from build123d import *

# Parameters (mm, degrees)
F0_W     = 3.8
F0_H     = 5
F0_W_2   = 4
F0_H_2   = 4
F0_R     = 2.5006647493
F0_R_2   = 4.8327220748
F0_R_3   = 3.906097333
F0_R_4   = 2.1231290944
F0_R_5   = 7.6831288046
F0_W_3   = 12
F0_H_3   = 6
F0_R_6   = 1.5
F1_DEPTH = 7
F2_SIZE  = 0.75


# Not quite as in the source:
# - a feature names something its author has since deleted; it is built from what else it names


with BuildPart() as f1:
    # F0 (on Top) → F1 (new body)
    with BuildSketch(Plane.XY):
        Polygon((0, 10.6260057762), (0, 15.6260057762), (-4, 15.6260057762), (-4, -26.3739942238), (0, -26.3739942238), (0, -22.3739942238), align=None)
        Polygon((8, 15.6260057762), (0, 15.6260057762), (0, 10.6260057762), (4.2, 10.6260057762), (8, 10.6260057762), align=None)
        with Locations((6.1, 8.1260057762)):
            Rectangle(F0_W, F0_H)
        with Locations((2, -24.3739942238)):
            Rectangle(F0_W_2, F0_H_2)
        Polygon((-4, -26.3739942238), (-4, 15.6260057762), (-42, 15.6260057762), (-42, 9.6260057762), (-54, 9.6260057762), align=None)
        with Locations((-21.8336265534, -6.3459714875)):
            Circle(F0_R, mode=Mode.SUBTRACT)
        with Locations((-12.1693955734, -9.9561735988)):
            Circle(F0_R_2, mode=Mode.SUBTRACT)
        with Locations((-28.6096986383, 0.2079327387)):
            Circle(F0_R, mode=Mode.SUBTRACT)
        with Locations((-36.4965982735, 7.095086854)):
            Circle(F0_R_3, mode=Mode.SUBTRACT)
        with Locations((-27.8876554221, 10.2054132149)):
            Circle(F0_R_4, mode=Mode.SUBTRACT)
        with Locations((-16.008509323, 5.6881718338)):
            Circle(F0_R_5, mode=Mode.SUBTRACT)
        with Locations((-48, 12.6260057762)):
            Rectangle(F0_W_3, F0_H_3)
        with Locations((-51, 12.6260057762)):
            Circle(F0_R_6, mode=Mode.SUBTRACT)
        with Locations((-45, 12.6260057762)):
            Circle(F0_R_6, mode=Mode.SUBTRACT)
    extrude(amount=F1_DEPTH)

    # F2
    f2_edges = [f1.edges().sort_by_distance(p)[0] for p in [
        (4.2, 5.626006, 3.5),
        (4, -22.373994, 3.5),
        (-17.002118, -9.956174, 0),
        (-31.110363, 0.207933, 0),
        (-40.402696, 7.095087, 7),
        (-40.402696, 7.095087, 0),
        (-30.010785, 10.205413, 0),
        (-23.691638, 5.688172, 0),
        (0, -5.873994, 0),
        (2.1, 10.626006, 0),
        (4.2, 8.126006, 0),
        (6.1, 5.626006, 0),
        (8, 10.626006, 0),
        (-23, 15.626006, 0),
        (-54, 12.626006, 0),
        (-29, -8.373994, 0),
        (0, -26.373994, 0),
        (4, -24.373994, 0),
        (2, -22.373994, 0),
        (-23, 15.626006, 7),
        (-54, 12.626006, 7),
        (-29, -8.373994, 7),
        (-30.010785, 10.205413, 7),
        (-31.110363, 0.207933, 7),
        (-23.691638, 5.688172, 7),
        (-17.002118, -9.956174, 7),
        (0, -26.373994, 7),
        (4, -24.373994, 7),
        (2, -22.373994, 7),
        (0, -5.873994, 7),
        (8, 10.626006, 7),
        (2.1, 10.626006, 7),
        (4.2, 8.126006, 7),
        (-24.334291, -6.345971, 7),
        (-24.334291, -6.345971, 0),
    ]]
    chamfer(f2_edges, length=F2_SIZE)


solid = f1.part
Input: part model. Units: mm. Frame: model coordinates. A direction names the side the tool comes from. Give positions to 0.01 mm unless a question says otherwise; leave off trailing zeros. Loops run counter-clockwise (first coordinate to the right, second up) from the corner with the lowest first, then second, coordinate; pieces in that order, holes last. Notation, with made-up numbers: (64, -28.75) - (82, -28.75) arc R22 ccw to (82, -16.75) - close; hole circle Ø2 at (46, 12.5). An arc over 180 degrees is marked (long way). Use CSV: the item, a comma, the result in double quotes. Start each with the question number.
Item 1: Line query: line 1 (X direction, y = -6, z = 5.5); line 2 (X direction, y = 9, z = 3); line 3 (Y direction, x = -15, z = 2.75). Output: solid intervals per line, ascending.
Item 2: Contact query for flat-ended pins moving along their axis: P1, Ø2, axis at y = 5.5, z = 1.5, coming from the -X side; P2, Ø1.6, axis at y = -10, z = 5, coming from the +X side; P3, Ø11, axis at x = -12.17, y = -9.96, coming from the -Z side; P4, Ø3.5, axis at x = -45, y = 12.63, coming from the +Z side. Output: stop coordinate, or through.
Item 3: Section D-D on x = -45. Return loops of the section in (y, z), then the cut area to 3 significant figures.
Item 4: Section B-B on z = 5. State how many separate pieces and enclosed holes the cut face has, then the cut area to 3 significant figures.
Item 5: Section C-C on y = -24. Return loops of the section in (x, z), then the cut area to 3 significant figures.
Item 6: Section A-A on x = 1.5. Return loops of the section in (y, z).
Item 7: Reachability of faces 1 (the flat face through (4.2, 8, 3)), 2 (the flat face through (4, -25, 3)), 3 (the flat face through (2, -22.374, 3)), 4 (the flat face through (2, 10.626, 3)) from +Z, -Z, +X, -X, +Y, -Y: full face, straight path, thin tool, end or side. Return the list, or none.
Ans:
1,line 1,"x = -32.3 to -24.31, -19.36 to -14.94, -9.39 to 0"
1,line 2,"x = -53.13 to -39.91, -33.09 to -29.64, -26.14 to -22.94, -9.08 to 0, 4.2 to 8"
1,line 3,"y = -18.45 to -13.87, -6.04 to -1.93, 13.3 to 15.63"
2,P1,"stops at x = -49.66"
2,P2,"stops at x = 0"
2,P3,"stops at z = 0.08"
2,P4,"stops at z = 7"
3,outline,"(3.15, 0.75) - (4.07, 0) - (11.13, 0) - (11.13, 7) - (4.07, 7) - (3.15, 6.25) - close; (14.13, 0) - (14.88, 0) - (15.63, 0.75) - (15.63, 6.25) - (14.88, 7) - (14.13, 7) - close"
3,area,"65.1 mm2"
4,separate pieces,"1"
4,enclosed holes,"8"
4,area,"1,070 mm2"
5,outline,"(-7.3, 0.75) - (-6.01, 0) - (3.25, 0) - (4, 0.75) - (4, 6.25) - (3.25, 7) - (-6.01, 7) - (-7.3, 6.25) - close"
5,area,"77.6 mm2"
6,outline,"(-26.37, 0.75) - (-25.62, 0) - (-23.12, 0) - (-22.37, 0.75) - (-22.37, 6.25) - (-23.12, 7) - (-25.62, 7) - (-26.37, 6.25) - close; (10.63, 0.75) - (11.38, 0) - (14.88, 0) - (15.63, 0.75) - (15.63, 6.25) - (14.88, 7) - (11.38, 7) - (10.63, 6.25) - close"
7,face 1,"+Z, -Z, -Y"
7,face 2,"+Z, -Z, +X, -Y"
7,face 3,"+Z, -Z, +X"
7,face 4,"+Z, -Z"
